The figure shows three views and two pictorial views of one solid part (mm, origin at its lowest corner). Answer the questions. A direction names the side the tool comes from. Coordinates: 2 decimals unless noted, no trailing zeros. Loops run counter-clockwise (first coordinate to the right, second up) from the corner with the lowest first, then second, coordinate; pieces in that order, holes last. Notation, with made-up numbers: (15.25, -5.5) -> (47.25, -5.5) arc R17 cw to (47.25, 17.5) -> close; hole circle Ø10 at (74.5, 42.25). An arc over 180 degrees is marked (long way). Answer in a Markdown table with one row per item.
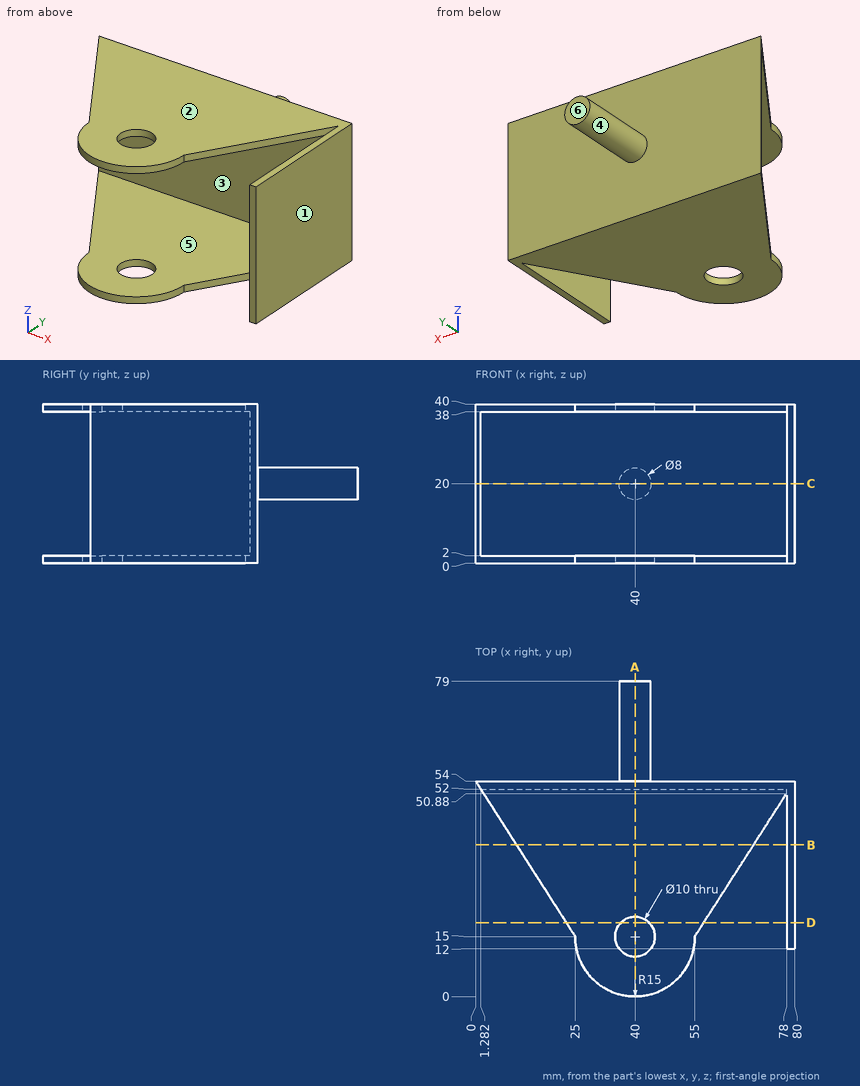
Item 1: Flat-ended cylindrical pins translate along their axes: pin 1 Ø18 at (x, z) = (51, 27.5) entering from -Y; pin 2 Ø2 at (y, z) = (9.5, 22.5) entering from -X; pin 3 Ø3 at (x, y) = (15.5, 30.5) entering from -Z; pin 4 Ø1 at (x, z) = (29, 26) entering from +Y. Find the tip coordinate at first contact, or state that the pin passes through.
Findings below:
| item | result |
|---|---|
| pin 1 | stops at y = 52 |
| pin 2 | passes through |
| pin 3 | stops at z = 0 |
| pin 4 | stops at y = 54 |
Item 2: A cutting plane is placed at A-A, the plane x = 40. Determine the outline of the cut face in (y, z), plus the area to 3 significant figures.
Findings below:
| item | result |
|---|---|
| outline | (0, 0) -> (10, 0) -> (10, 2) -> (0, 2) -> close; (0, 38) -> (10, 38) -> (10, 40) -> (0, 40) -> close; (20, 0) -> (54, 0) -> (54, 16) -> (79, 16) -> (79, 24) -> (54, 24) -> (54, 40) -> (20, 40) -> (20, 38) -> (52, 38) -> (52, 2) -> (20, 2) -> close |
| area | 448 mm2 |
Item 3: A cutting plane is placed at C-C, the plane z = 20. Determine the outline of the cut face in (x, y).
Findings below:
| item | result |
|---|---|
| outline | (0, 54) -> (1.28, 52) -> (78, 52) -> (78, 12) -> (80, 12) -> (80, 54) -> (44, 54) -> (44, 79) -> (36, 79) -> (36, 54) -> close |
Item 4: A cutting plane is placed at B-B, the plane y = 38. Determine the outline of the cut face in (x, z).
Findings below:
| item | result |
|---|---|
| outline | (10.26, 0) -> (69.74, 0) -> (69.74, 2) -> (10.26, 2) -> close; (10.26, 38) -> (69.74, 38) -> (69.74, 40) -> (10.26, 40) -> close; (78, 0) -> (80, 0) -> (80, 40) -> (78, 40) -> close |
Item 5: A cutting plane is placed at D-D, the plane y = 18.5. Determine the outline of the cut face in (x, z), plus the area to 3 significant figures.
Findings below:
| item | result |
|---|---|
| outline | (22.76, 0) -> (36.43, 0) -> (36.43, 2) -> (22.76, 2) -> close; (22.76, 38) -> (36.43, 38) -> (36.43, 40) -> (22.76, 40) -> close; (43.57, 0) -> (57.24, 0) -> (57.24, 2) -> (43.57, 2) -> close; (43.57, 38) -> (57.24, 38) -> (57.24, 40) -> (43.57, 40) -> close; (78, 0) -> (80, 0) -> (80, 40) -> (78, 40) -> close |
| area | 189 mm2 |
Item 6: Determine the mould class of the marked faces 1, 2 and 3 for opening direction Z: +Z half, -Z half, draft (parallel to the pull), parting line (faces both ways), or undercut.
Findings below:
| item | result |
|---|---|
| face 1 | draft |
| face 2 | +Z half |
| face 3 | undercut |
Item 7: Find the intervals of material crossed by probe 1 along X at (y, z) = (15, 1.5); probe 2 along Z at (x, y) = (48.5, 48); probe 3 along X at (y, z) = (26.5, 19.5), in increasing order.
Findings below:
| item | result |
|---|---|
| probe 1 | x = 25 to 35, 45 to 55, 78 to 80 |
| probe 2 | z = 0 to 2, 38 to 40 |
| probe 3 | x = 78 to 80 |
Item 8: A tool of negligible diameter and unlimited length cuts with its end or side. For the marked faces 4, 5 and 6, from which of +Z, -Z, +X, -X, +Y, -Y can it reach the whole face along a straight path? Write none if from no direction.
Findings below:
| item | result |
|---|---|
| face 4 | +Y |
| face 5 | -X, -Y |
| face 6 | +Z, -Z, +X, -X, +Y |
